Could you check a few things on this model? Use its own coordinates, in mm. A direction names the side the tool comes from. Coordinates: 2 decimals unless noted, no trailing zeros. Order: outer loops, then holes, each group sorted by start corner. A loop starts at its lowest first (then second) coordinate and runs counter-clockwise, first axis right, second up. Notation, with made-up numbers: (-0.75, 73.5) - (22.25, 73.5) arc R34 ccw to (22.25, 111.5) - close; hole circle Ø2 at (48, -13). An arc over 180 degrees is marked (long way). Answer as a JSON object with one key per item and string values. Group by question number.
(1) We'd pull the mould along Z, two halves only. Please class faces 1 (the flat face through (750, 18, 5)), 2 (the cylindrical face through (706.864, -319.464, -304.248)), 3 (the flat face through (-10, 18, -375)): pulls with the +Z half, pulls with the -Z half, needs draft (parallel to the pull), parting line crosses it, or undercut.
(2) Which directions (+Z, -Z, +X, -X, +Y, -Y) give clear straight access to the entire face, cutting with the end or side of a thin tool? Please do faces 4 (the flat face through (-10, 36.5, -5)), 5 (the cylindrical face through (706.864, -319.464, 304.248)).
(3) Imagine slicing it at B-B, the plane y = -465. Write out the boundary of the cut face in (x, z).
(4) Imagine slicing it at A-A, the plane z = -315. Write out the boundary of the cut face in (x, y), and give its area (3 significant figures).
(5) Imagine slicing it at D-D, the plane z = 33. Write out the boundary of the cut face in (x, y).
(6) Please list where these lines run through material, in increasing order: probe 1 along Y at (x, z) = (-363, -320.5); probe 2 along X at (y, z) = (-117, 306).
(7) Imagine slicing it at C-C, the plane x = -114.5. Write out the boundary of the cut face in (y, z), and give its area (3 significant figures).
from build123d import *

# Parameters (mm, degrees)
SKETCH1_W           = 1500
SKETCH1_H           = 750
BOSS_EXTRUDE1_DEPTH = 36.5
SKETCH2_R           = 20
BOSS_EXTRUDE2_DEPTH = 648


with BuildPart() as part:
    # Sketch1 → Boss-Extrude1 (new body)
    with BuildSketch(Plane(origin=(0, 0, 0), x_dir=(1, 0, 0), z_dir=(0, 1, 0))):
        Rectangle(SKETCH1_W, SKETCH1_H)
    extrude(amount=BOSS_EXTRUDE1_DEPTH)

    # Sketch2 → Boss-Extrude2 (add)
    with BuildSketch(Plane.XZ):
        with Locations(Location((690, 315, 0), (0, 0, 270))):
            Circle(SKETCH2_R)
    boss_extrude2 = extrude(amount=BOSS_EXTRUDE2_DEPTH)

    # Mirror1: Boss-Extrude2 across plane
    add(boss_extrude2.mirror(Plane.XY))


solid = part.part
Result set:
{
 "1": {"face 1": "needs draft", "face 2": "undercut", "face 3": "pulls with the -Z half"},
 "2": {"face 4": "+Z, -Z, +X, -X, +Y", "face 5": "-Y"},
 "3": {"outline": "circle Ø40 at (690, -315); circle Ø40 at (690, 315)"},
 "4": {"outline": "(-750, 0) - (670, 0) - (670, -648) - (710, -648) - (710, 0) - (750, 0) - (750, 36.5) - (-750, 36.5) - close", "area": "80,700 mm^2"},
 "5": {"outline": "(-750, 0) - (750, 0) - (750, 36.5) - (-750, 36.5) - close"},
 "6": {"probe 1": "y = 0 to 36.5", "probe 2": "x = 672.14 to 707.86"},
 "7": {"outline": "(0, -375) - (36.5, -375) - (36.5, 375) - (0, 375) - close", "area": "27,400 mm^2"}
}
